Build history of the part. All positions in model axes, mm. A direction names the side the tool comes from. Round coordinates to 2 decimals unless told otherwise and drop trailing zeros. Write each loop counter-clockwise with the first axis right and the second up, starting at its lowest first coordinate (ties: lowest second). Pieces come first, ordered by that corner, then holes. Notation, with made-up numbers: M 87.25,80 L 109.25,80 A21 cw 109.25,110 Z; hole C 56,59 d9. An arc over 180 degrees is marked long. Write item = value, one per line. Start each with the question number.
Q1. Band-saw the part on A-A on z = 2.25. Write the cut outline in (x, y).
Q2. Band-saw the part on B-B on z = -3.75. Write the cut outline in (x, y), plus the area to 3 significant figures.
Q3. Drop flat-ended pins along their axis: P1, Ø2.5, axis at x = 7, z = 5, coming from the +Y side; P2, Ø1.9, axis at x = 1.5, y = 0.5, coming from the +Z side; P3, Ø2, axis at x = 7, z = 16.5, coming from the -Y side. Give the stop position or say it passes through.
Q4. Band-saw the part on C-C on x = 7.1. State how many separate pieces and enclosed holes the cut face has, plus the area to 3 significant figures.
Q5. Band-saw the part on D-D on y = -0.75. Write the cut outline in (x, z).
Q6. Probe L1, parallel to Z at x = 7.1, y = 1.9; L2, parallel to Z at x = -1.75, y = 2; L3, parallel to Y at x = 0, z = 2. List the from-to ranges inside material, lowest first.
Q7. Pull direction Z, two halves, no side cores. Call faces 5 (the flat face through (5, 2.1, 2)), 6 (the flat face through (6, 1, -7.75)), 7 (the flat face through (3.1, 1, 10)): released by +Z, released by -Z, zero draft, split by the parting line, or undercut.
Q8. Tool access for faces 1 (the flat face through (3.1, 1, 23)), 2 (the flat face through (-2.7, 2.1, 15.7)), 3 (the flat face through (2, 0, 12)), 4 (the flat face through (7, 2.1, 20)): list every direction of +Z, -Z, +X, -X, +Y, -Y with a clear straight run to the whole face (end or side of a thin tool).
```python
from build123d import *

# Parameters (mm, degrees)
SKETCH2_R           = 1.6
BOSS_EXTRUDE1_DEPTH = 7.5
SKETCH4_W           = 8
SKETCH4_H           = 1.5
BOSS_EXTRUDE3_DEPTH = 4.5
SKETCH5_R           = 1.6
BOSS_EXTRUDE4_DEPTH = 7.5
SKETCH6_W           = 8
SKETCH6_H           = 1.5
BOSS_EXTRUDE5_DEPTH = 7.75
SKETCH7_W           = 8
SKETCH7_H           = 1.5
BOSS_EXTRUDE6_DEPTH = 7.75
SKETCH8_W           = 0.75
SKETCH8_H           = 0.5
CUT_EXTRUDE1_DEPTH  = 9
SKETCH9_R           = 1.1
CUT_EXTRUDE2_DEPTH  = 3.5
CHAMFER1_SIZE       = 1.1
FILLET1_R           = 3


with BuildPart() as part:
    # Sketch2 → Boss-Extrude1 (new body)
    with BuildSketch(Plane.XY):
        with BuildLine():
            Line((3.1, 2.1), (11.1, 2.1))
            Line((11.1, 2.1), (11.1, 0.6))
            Line((11.1, 0.6), (3.1, 0.6))
            Line((3.1, 0.6), (3.1, 0))
            ThreePointArc((3.1, 0), (0, -3.1), (-3.1, 0))
            Line((-3.1, 0), (-3.1, 2.1))
            Line((-3.1, 2.1), (-2.28035085, 2.1))
            ThreePointArc((-2.28035085, 2.1), (-1.24498996, 2.839013913), (0, 3.1))
            Line((0, 3.1), (3.1, 3.1))
            Line((3.1, 3.1), (3.1, 2.1))
        make_face()
        Circle(SKETCH2_R, mode=Mode.SUBTRACT)
    extrude(amount=BOSS_EXTRUDE1_DEPTH)

    # Sketch4 → Boss-Extrude3 (add)
    with BuildSketch(Plane.XY.offset(7.5)):
        with Locations((7.1, 1.35)):
            Rectangle(SKETCH4_W, SKETCH4_H)
    extrude(amount=BOSS_EXTRUDE3_DEPTH)

    # Sketch5 → Boss-Extrude4 (add)
    with BuildSketch(Plane.XY.offset(12)):
        with BuildLine():
            Line((11.1, 0.6), (11.1, 2.1))
            Line((11.1, 2.1), (3.1, 2.1))
            Line((3.1, 2.1), (3.1, 3.1))
            Line((3.1, 3.1), (0, 3.1))
            ThreePointArc((0, 3.1), (-1.24498996, 2.839013913), (-2.28035085, 2.1))
            Line((-2.28035085, 2.1), (-3.1, 2.1))
            Line((-3.1, 2.1), (-3.1, 0))
            ThreePointArc((-3.1, 0), (0, -3.1), (3.1, 0))
            Line((3.1, 0), (3.1, 0.6))
            Line((3.1, 0.6), (11.1, 0.6))
        make_face()
        Circle(SKETCH5_R, mode=Mode.SUBTRACT)
    extrude(amount=BOSS_EXTRUDE4_DEPTH)

    # Sketch6 → Boss-Extrude5 (add)
    with BuildSketch(Plane.XY.offset(19.5)):
        with Locations((7.1, 1.35)):
            Rectangle(SKETCH6_W, SKETCH6_H)
    extrude(amount=BOSS_EXTRUDE5_DEPTH)

    # Sketch7 → Boss-Extrude6 (add)
    with BuildSketch(Plane(origin=(0, 0, 0), x_dir=(-1, 0, 0), z_dir=(0, 0, -1))):
        with Locations((-7.1, 1.35)):
            Rectangle(SKETCH7_W, SKETCH7_H)
    extrude(amount=BOSS_EXTRUDE6_DEPTH)

    # Sketch8 → Cut-Extrude1 (cut, through all)
    with BuildSketch(Plane.ZY.offset(-3.1)):
        with Locations((11.625, 1.85)):
            Rectangle(SKETCH8_W, SKETCH8_H)
    extrude(amount=-CUT_EXTRUDE1_DEPTH, mode=Mode.SUBTRACT)

    # Sketch9 → Cut-Extrude2 (cut, through all)
    with BuildSketch(Plane.XZ.offset(-0.6)):
        with Locations((7.1, 23.25)):
            Circle(SKETCH9_R)
        with Locations((7.1, 17.25)):
            Circle(SKETCH9_R)
        with Locations((7.1, 2.25)):
            Circle(SKETCH9_R)
        with Locations((7.1, -3.75)):
            Circle(SKETCH9_R)
    extrude(amount=-CUT_EXTRUDE2_DEPTH, mode=Mode.SUBTRACT)

    # Chamfer1
    chamfer1_edges = [part.edges().sort_by_distance(p)[0] for p in [
        (6, 0.6, 23.25),
        (6, 0.6, 17.25),
        (6, 0.6, 2.25),
        (6, 0.6, -3.75),
    ]]
    chamfer(chamfer1_edges, length=CHAMFER1_SIZE)

    # Fillet1
    fillet1_edges = [part.edges().sort_by_distance(p)[0] for p in [
        (11.1, 1.35, 27.25),
        (11.1, 1.35, -7.75),
    ]]
    fillet(fillet1_edges, radius=FILLET1_R)


solid = part.part
```
Conclusion:
q1.outline = M -3.1,0 A3.1 ccw 3.1,0 L 3.1,0.6 L 4.9,0.6 L 6,1.7 L 6,2.1 L 3.1,2.1 L 3.1,3.1 L 0,3.1 A3.1 ccw -2.28,2.1 L -3.1,2.1 Z; M 8.2,1.7 L 9.3,0.6 L 11.1,0.6 L 11.1,2.1 L 8.2,2.1 Z; hole C 0,0 d3.2
q2.outline = M 3.1,0.6 L 4.9,0.6 L 6,1.7 L 6,2.1 L 3.1,2.1 Z; M 8.2,1.7 L 9.3,0.6 L 11.1,0.6 L 11.1,2.1 L 8.2,2.1 Z
q2.area = 7.49 mm^2
q3.P1 = 2.1
q3.P2 = 19.5
q3.P3 = 1.04
q4.separate_pieces = 5
q4.enclosed_holes = 0
q4.area = 34.1 mm^2
q5.outline = M -3.01,0 L -1.41,0 L -1.41,7.5 L -3.01,7.5 Z; M -3.01,12 L -1.41,12 L -1.41,19.5 L -3.01,19.5 Z; M 1.41,0 L 3.01,0 L 3.01,7.5 L 1.41,7.5 Z; M 1.41,12 L 3.01,12 L 3.01,19.5 L 1.41,19.5 Z
q6.L1 = -7.75 to -4.85, -2.65 to 1.15, 3.35 to 11.25, 12 to 16.15, 18.35 to 22.15, 24.35 to 27.25
q6.L2 = 0 to 7.5, 12 to 19.5
q6.L3 = -3.1 to -1.6, 1.6 to 3.1
q7.face_5 = zero draft
q7.face_6 = released by -Z
q7.face_7 = undercut
q8.face_1 = +Z, -X, +Y, -Y
q8.face_2 = +Z, -Z, -X, +Y
q8.face_3 = -X, +Y
q8.face_4 = +Z, -Z, +X, +Y
